Autodesk Inventor part; units mm, degrees
ref_plane "Work Plane1" through (0, -215.9, -38.1) normal (0, 0, 1) x (1, 0, 0)
ref_plane "YZ Plane" through (0, 0, 0) normal (1, 0, 0) x (0, 1, 0)
ref_plane "XZ Plane" through (0, 0, 0) normal (0, 1, 0) x (-1, 0, 0)
sketch "Sketch1" plane through (0, 0, 0) normal (1, 0, 0) x (0, 1, 0)
  line L0 (0, 0) -> (-228.6, 0)
  line L1 (-228.6, 0) -> (-228.6, -12.7)
  line L2 (-228.6, -12.7) -> (0, -12.7)
  line L3 (0, -12.7) -> (0, 0)
  line L4 (0, -12.7) -> (-88.9, -12.7)
  line L5 (-88.9, -63.5) -> (0, -63.5)
  line L6 (0, -63.5) -> (-228.6, -63.5)
  line L7 (-228.6, -63.5) -> (-228.6, -76.2)
  line L8 (-228.6, -76.2) -> (0, -76.2)
  line L9 (0, -76.2) -> (0, -63.5)
  line L10 (-228.6, 0) -> (-215.9, 0)
  line L11 (-215.9, 0) -> (-215.9, -76.2)
  line L12 (-215.9, -76.2) -> (-228.6, -76.2)
  line L13 (-228.6, -76.2) -> (-228.6, 0)
  dimension "d1" = 12.7
  dimension "d4" = 12.7
  dimension "d63" = 12.7
  dimension "d64" = 228.6
  dimension "d65" = 228.6
  dimension "d66" = 50.8
extrude "Extrusion1" add sketch "Sketch1" along normal blind 25.4
sketch "Sketch3" plane through (0, -228.6, -76.2) normal (0, 0, -1) x (-1, 0, 0)
  line L0 (0, 0) -> (0, 228.6)
  line L1 (0, 228.6) -> (-25.4, 228.6)
  line L2 (-25.4, 0) -> (-25.4, 228.6)
  line L3 (0, 0) -> (-25.4, 0)
  point P0 (0, 228.6)
  point P1 (-12.7, 31.75)
  dimension "d18" = 25.4
  dimension "d19" = 12.7
  dimension "d20" = 31.75
hole "Hole2" at (12.7, -196.85, -76.2) direction (0, 0, 1) diameter 11.9888 end through all
sketch "Sketch5" plane through (25.4, 0, 0) normal (1, 0, 0) x (0, 0, -1)
  line L0 (0, 0) -> (12.7, 0)
  line L1 (12.7, 0) -> (12.7, -25.4)
  line L2 (12.7, -25.4) -> (0, -25.4)
  line L3 (0, -25.4) -> (0, 0)
  line L4 (0, 0) -> (0, -228.6)
  line L5 (12.7, 0) -> (0, 0)
  dimension "d39" = 12.7
  dimension "d67" = 25.4
  dimension "d68" = 0
  dimension "d69" = 0
extrude "Extrusion2" add sketch "Sketch5" along normal blind 247.65
sketch "Sketch9" plane through (25.4, 0, 0) normal (1, 0, 0) x (0, 0, -1)
  line L0 (12.7, -215.9) -> (12.7, -25.4)
  line L1 (0, -95.25) -> (12.7, -95.25)
  line L2 (12.7, -95.25) -> (12.7, -120.65)
  line L3 (12.7, -120.65) -> (0, -120.65)
  line L4 (0, -120.65) -> (0, -95.25)
  line L5 (0, -25.4) -> (0, -228.6)
  line L6 (0, -25.4) -> (12.7, -25.4)
  point P0 (0, 0)
  dimension "d81" = 25.4
  dimension "d83" = 12.7
  dimension "d84" = 12.7
  dimension "d85" = 69.85
extrude "Extrusion3" add sketch "Sketch9" along normal blind 76.2 contours L3 L4 L1 L0
sketch "Sketch8" plane through (0, -215.9, -12.7) normal (0, 0, -1) x (-1, 0, 0)
  line L0 (-273.05, 190.5) -> (-273.05, 215.9)
  line L1 (0, 215.9) -> (-273.05, 215.9)
  point P0 (-254, 203.2)
  dimension "d70" = 19.05
  dimension "d71" = 25.4
  dimension "d72" = 12.7
hole "Hole6" at (254, -12.7, -12.7) direction (0, 0, 1) diameter 12.7 end through all
ref_plane "Work Plane1" through (0, -215.9, -38.1) normal (0, 0, 1) x (1, 0, 0)
mirror "Mirror1" about plane through (0, -215.9, -38.1) normal (0, 0, 1) of "Extrusion3"
sketch "Sketch10" plane through (0, -228.6, 0) normal (0, 0, 1) x (1, 0, 0)
  line L0 (25.4, 133.35) -> (101.6, 133.35)
  line L1 (25.4, 107.95) -> (101.6, 107.95)
  line L2 (101.6, 133.35) -> (101.6, 107.95)
  point P0 (0, 228.6)
  point P1 (88.9, 120.65)
  dimension "d89" = 25.4
  dimension "d90" = 12.7
  dimension "d91" = 12.7
hole "Hole7" at (88.9, -107.95, 0) direction (0, 0, -1) diameter 12.827 end through all
sketch "Sketch11" plane through (0, -215.9, -63.5) normal (0, 0, 1) x (1, 0, 0)
  line L0 (0, 215.9) -> (25.4, 215.9)
  line L1 (25.4, 215.9) -> (25.4, 120.65)
  line L2 (0, 215.9) -> (25.4, 215.9)
  line L3 (25.4, 215.9) -> (25.4, 203.2)
  line L4 (25.4, 203.2) -> (0, 203.2)
  line L5 (0, 203.2) -> (0, 215.9)
  dimension "d99" = 12.7
extrude "Extrusion4" add sketch "Sketch11" along normal up to surface (50.8 mm away)
sketch "Sketch12" plane through (25.4, 0, 0) normal (1, 0, 0) x (0, 0, -1)
  line L0 (76.2, -228.6) -> (76.2, 0)
  line L1 (76.2, -133.35) -> (63.5, -133.35)
  line L2 (63.5, -12.7) -> (63.5, -215.9)
  line L3 (76.2, -120.65) -> (63.5, -120.65)
  line L4 (12.7, -215.9) -> (12.7, -12.7)
  line L5 (0, 0) -> (0, -228.6)
  line L6 (76.2, -120.65) -> (63.5, -120.65)
  line L7 (63.5, -120.65) -> (63.5, -215.9)
  line L8 (63.5, -215.9) -> (12.7, -215.9)
  line L9 (12.7, -215.9) -> (12.7, -120.65)
  line L10 (12.7, -120.65) -> (0, -120.65)
  line L11 (0, -120.65) -> (0, -228.6)
  line L12 (0, -228.6) -> (76.2, -228.6)
  line L13 (76.2, -228.6) -> (76.2, -120.65)
  line L14 (12.7, -215.9) -> (0, -215.9)
  dimension "d102" = 12.7
extrude "Extrusion5" cut sketch "Sketch12" against normal blind 50.8 contours L12 L5 L14 L8 L2 L1 L0
sketch "Sketch13" plane through (0, 0, 0) normal (0, 0, 1) x (1, 0, 0)
  circle A0 centre (12.7, -196.85) radius 5.9944
  point P0 (0, 0)
  point P1 (6.2738, -189.103)
  point P2 (19.7104, -181.356)
  point P3 (19.7104, -212.344)
  point P4 (6.2738, -204.597)
  dimension "d105" = 7.747
  dimension "d106" = 6.4262
  dimension "d107" = 7.0104
  dimension "d108" = 15.494
  dimension "d109" = 15.494
  dimension "d110" = 7.0104
  dimension "d111" = 7.747
  dimension "d112" = 6.4262
hole "Hole8" at (6.2738, -189.103, 0) at (19.7104, -181.356, 0) at (19.7104, -212.344, 0) at (6.2738, -204.597, 0) direction (0, 0, -1) diameter 3.175 end through all
equation "\"d4\" = d1"
equation "\"d65\" = d64"
equation "\"d84\" = d83"
properties part number "shooter" material "Aluminum 6061"
CAD build for the part. Positions are in the model's coordinates, mm. A direction names the side the tool comes from. Round coordinates to 2 decimals unless told otherwise and drop trailing zeros. Loops run counter-clockwise (first coordinate to the right, second up) from the corner with the lowest first, then second, coordinate; pieces in that order, holes last.
(1) Cut at C-C (x = 12.7). Give the cut face in (y, z).
(2) Cut at D-D (z = -68). Give the cut face in (x, y).
(3) Which spindle directions (+Z, -Z, +X, -X, +Y, -Y) get a long thin tool onto all of the face, cutting with end or side? Do faces 4 (the flat face through (63, -95.25, -70)), 5 (the flat face through (13, -133.35, -70)), 6 (the flat face through (25.4, -169, -6)), 7 (the flat face through (75, -99, -12.7)), 8 (the flat face through (25.4, -30, -68)). Say none if no direction does.
(4) Cut at B-B (y = -89.5). Give the cut face in (x, z), plus the area to 3 significant figures.
(5) Cut at A-A (x = 88.9). Give the cut face in (y, z).
(6) Drop flat-ended pins along their axis: pin 1 (6.5 mm diameter, centred on x = 56.5, z = -70.5, fed in from -Y); pin 2 (12 mm diameter, centred on x = 75.5, y = -125, fed in from +Z); pin 3 (2.5 mm diameter, centred on x = 6.27, y = -189.1, fed in from +Z); pin 4 (3 mm diameter, centred on y = -155.5, z = -8, fed in from +X). Give the stop position or say it passes through.
(7) Two-plate mould, pull along Z, no slides. Class faces 1 (the flat face through (85, -100, 0)), 2 (the flat face through (63, -120.65, -6)), 3 (the flat face through (28, -99, -63.5)): +Z half, -Z half, draft (parallel to the pull), parting line (faces both ways), or undercut.
(8) Wall check: line 1 along X through (y, z) = (-12.7, -7.5); line 2 along X through (y, z) = (-107, -73); line 3 along Y through (x, z) = (12.7, -8.5). Give the ranges that are in metal, low to high.
Findings below:
1. outline: (-215.9, -12.7) - (-202.84, -12.7) - (-202.84, 0) - (-215.9, 0) - close; (-190.86, -12.7) - (-12.7, -12.7) - (-12.7, -63.5) - (-133.35, -63.5) - (-133.35, -76.2) - (0, -76.2) - (0, 0) - (-190.86, 0) - close
2. outline: (0, -133.35) - (25.4, -133.35) - (25.4, -120.65) - (101.6, -120.65) - (101.6, -95.25) - (25.4, -95.25) - (25.4, 0) - (0, 0) - close; hole circle Ø12.83 at (88.9, -107.95)
3. face 4: +Z, -Z, +X, +Y
3. face 5: -Z, +X, -X, -Y
3. face 6: +Z, -Z, +X, -Y
3. face 7: +X, -Y
3. face 8: -Z, +X, +Y
4. outline: (0, -76.2) - (25.4, -76.2) - (25.4, -63.5) - (0, -63.5) - close; (0, -12.7) - (25.4, -12.7) - (25.4, 0) - (0, 0) - close
4. area: 645 mm2
5. outline: (-120.65, -76.2) - (-114.36, -76.2) - (-114.36, -63.5) - (-120.65, -63.5) - close; (-120.65, -12.7) - (-114.36, -12.7) - (-114.36, 0) - (-120.65, 0) - close; (-101.54, -76.2) - (-95.25, -76.2) - (-95.25, -63.5) - (-101.54, -63.5) - close; (-101.54, -12.7) - (-95.25, -12.7) - (-95.25, 0) - (-101.54, 0) - close; (-25.4, -12.7) - (0, -12.7) - (0, 0) - (-25.4, 0) - close
6. pin 1: stops at y = -120.65
6. pin 2: stops at z = 0
6. pin 3: passes through
6. pin 4: stops at x = 25.4
7. face 1: +Z half
7. face 2: draft
7. face 3: undercut
8. line 1: x = 0 to 247.65, 260.35 to 273.05
8. line 2: x = 0 to 82.56, 95.24 to 101.6
8. line 3: y = -215.9 to -202.84, -190.86 to 0
